from build123d import *

# Parameters (mm, degrees)
BOSS_EXTRUDE2_DEPTH = 3.175


with BuildPart() as part:
    # Sketch2 → Boss-Extrude2 (new body)
    with BuildSketch(Plane(origin=(0, 0, 0), x_dir=(0, 0, -1), z_dir=(1, 0, 0))):
        Polygon((0, 101.6), (0, 76.2), (3.175, 76.2), (3.175, 25.4), (0, 25.4), (0, 0), (12.7, 0), (12.7, 95.25), (15.875, 95.25), (15.875, 0), (25.4, 0), (25.4, 95.25), (28.575, 95.25), (28.575, 0), (38.1, 0), (38.1, 95.25), (41.275, 95.25), (41.275, 0), (50.8, 0), (50.8, 95.25), (53.975, 95.25), (53.975, 0), (63.5, 0), (63.5, 95.25), (66.675, 95.25), (66.675, 0), (76.2, 0), (76.2, 95.25), (79.375, 95.25), (79.375, 0), (88.9, 0), (88.9, 95.25), (92.075, 95.25), (92.075, 0), (101.6, 0), (101.6, 95.25), (104.775, 95.25), (104.775, 0), (114.3, 0), (114.3, 95.25), (117.475, 95.25), (117.475, 0), (127, 0), (127, 95.25), (130.175, 95.25), (130.175, 0), (139.7, 0), (139.7, 95.25), (142.875, 95.25), (142.875, 0), (159.512, 0), (159.512, 25.4), (162.687, 25.4), (162.687, 76.2), (159.512, 76.2), (159.512, 101.6), (149.225, 101.6), (149.225, 6.35), (146.05, 6.35), (146.05, 101.6), (136.525, 101.6), (136.525, 6.35), (133.35, 6.35), (133.35, 101.6), (123.825, 101.6), (123.825, 6.35), (120.65, 6.35), (120.65, 101.6), (111.125, 101.6), (111.125, 6.35), (107.95, 6.35), (107.95, 101.6), (98.425, 101.6), (98.425, 6.35), (95.25, 6.35), (95.25, 101.6), (85.725, 101.6), (85.725, 6.35), (82.55, 6.35), (82.55, 101.6), (73.025, 101.6), (73.025, 6.35), (69.85, 6.35), (69.85, 101.6), (60.325, 101.6), (60.325, 6.35), (57.15, 6.35), (57.15, 101.6), (47.625, 101.6), (47.625, 6.35), (44.45, 6.35), (44.45, 101.6), (34.925, 101.6), (34.925, 6.35), (31.75, 6.35), (31.75, 101.6), (25.358279829, 101.6), (22.225, 101.6), (22.225, 6.35), (19.05, 6.35), (19.05, 101.6), align=None)
    extrude(amount=BOSS_EXTRUDE2_DEPTH)


solid = part.part
The listing builds one solid part. Answer for the finished solid, in the listing's coordinates (mm). A direction names the side the tool comes from. Coordinates: 2 decimals unless noted, no trailing zeros. Use CSV: the item, a comma, the result in double quotes.
Q1. A tool of negligible diameter and unlimited length cuts with its end or side. For faces 4 (the flat face through (2, 95.25, -27)), 5 (the flat face through (2, 13, -159.512)), 6 (the flat face through (2, 0, -122)), 7 (the flat face through (2, 55, -136.525)), from which of +Z, -Z, +X, -X, +Y, -Y can it reach the whole face along a straight path? Write none if from no direction.
Here are the results:
face 4,"+X, -X, -Y"
face 5,"-Z, +X, -X, -Y"
face 6,"+Z, -Z, +X, -X, -Y"
face 7,"+X, -X, +Y"
Q2. Determine the mould class of faces 1 (the flat face through (2, 101.6, -27)), 2 (the flat face through (2, 6.35, -46)), 3 (the flat face through (2, 51, -3.175)) for opening direction Z: pulls with the +Z half, pulls with the -Z half, needs draft (parallel to the pull), parting line crosses it, or undercut.
Here are the results:
face 1,"needs draft"
face 2,"undercut"
face 3,"pulls with the +Z half"
Q3. Given pin 1 Ø12 at (y, z) = (39.5, -49.5) entering from -X; pin 2 Ø1 at (x, z) = (1.5, -65) entering from -Y; pin 3 Ø1 at (x, z) = (2, -58) entering from +Y; pin 4 Ø2 at (y, z) = (64.5, -46.5) entering from +X, each flat-ended and moving along its own axis, determine where each tip first touches the part or whether it passes through.
Here are the results:
pin 1,"x = 0"
pin 2,"y = 95.25"
pin 3,"y = 6.35"
pin 4,"through"
Q4. Section A-A (y = 60) is taken. Give the number of separate pieces and of enclosed holes in the cut face, then the cut area to 3 significant figures.
Here are the results:
separate pieces,"23"
enclosed holes,"0"
area,"285 mm2"
Q5. Straight lines are drawn through the part: L1, parallel to Y at x = 0.4, z = -123; L2, parallel to Y at x = 2.1, z = -115. For each, find the intervals that lie inside material, in ascending order.
Here are the results:
L1,"0 to 6.35"
L2,"95.25 to 101.6"
